Here's how the part is built. I have some questions about the finished solid (model axes, mm). A direction names the side the tool comes from. Coordinates: 2 decimals unless noted, no trailing zeros. Order: outer loops, then holes, each group sorted by start corner. A loop starts at its lowest first (then second) coordinate and runs counter-clockwise, first axis right, second up. Notation, with made-up numbers: (-17, -28.75) - (26, -28.75) arc R27 cw to (26, 1.25) - close; hole circle Ø6 at (-33.75, 17.25). An arc over 180 degrees is marked (long way). Answer as CSV lines item,"result". Start each with the question number.
Item 1: I'm going to push flat-ended pins straight in: pin 1 (2 mm diameter, centred on y = 12, z = 5, fed in from +X); pin 2 (4.5 mm diameter, centred on x = 19.5, z = 6, fed in from -Y); pin 3 (2 mm diameter, centred on x = 19, z = 4, fed in from +Y). Where does each tip first touch, or does it pass through?
Item 2: Imagine slicing it at D-D on x = -3. List the corners of the cut face in (y, z) for me, and give its area (3 significant figures).
Item 3: Imagine slicing it at A-A on x = 3. List the corners of the cut face in (y, z) for me, and give its area (3 significant figures).
Item 4: Imagine slicing it at C-C on z = 10.5. List the corners of the cut face in (x, y) for me, and give its area (3 significant figures).
Item 5: On a 3-axis mill with a long thin cutter (end or side, diameter ignored), from which of +Z, -Z, +X, -X, +Y, -Y can I reach the whole of each face in a straight line? I mean faces 1 (the face through (17, 8.069, 6)), 2 (the face through (-8, 10.569, 7)), 3 (the face through (-9, 9, 4.9)). Say none if no direction works.
Item 6: I need wall thicknesses on line 1 (Y direction, x = -2, z = 3); line 2 (X direction, y = 4, z = 7.25); line 3 (Y direction, x = -7.5, z = 1.75). Which ranges of each line are inside material? Lowest first, please.
Item 7: Imagine slicing it at B-B on y = 7. List the corners of the cut face in (x, z) for me, and give its area (4 significant figures).
from build123d import *

# Parameters (mm, degrees)
SKETCH2_W                = 22.5
SKETCH2_H                = 22.7
BOSS_EXTRUDE1_DEPTH      = 11.8
SKETCH3_R                = 5.9
BOSS_EXTRUDE2_DEPTH      = 4
SKETCH4_R                = 2.3
BOSS_EXTRUDE3_DEPTH      = 3.2
BOSS_EXTRUDE4_DEPTH      = 4
BOSS_EXTRUDE4_DEPTH_BACK = 26.5
SKETCH5_W                = 11.8
SKETCH5_H                = 2.5
CUT_EXTRUDE1_REACH       = 32.014


with BuildPart() as part:
    # Sketch2 → Boss-Extrude1 (new body)
    with BuildSketch(Plane.XY):
        with Locations((5.317300213, 3.518634424)):
            Rectangle(SKETCH2_W, SKETCH2_H)
    extrude(amount=BOSS_EXTRUDE1_DEPTH)

    # Sketch3 → Boss-Extrude2 (add)
    with BuildSketch(Plane(origin=(0, 14.868634424, 0), x_dir=(1, 0, 0), z_dir=(0, 1, 0))):
        with Locations((-0.032699787, -5.9)):
            Circle(SKETCH3_R)
        with BuildLine():
            ThreePointArc((5.31155509, -3.400212046), (5.726688366, -4.619590646), (5.867300213, -5.9))
            ThreePointArc((5.867300213, -5.9), (5.726688366, -7.180409354), (5.31155509, -8.399787954))
            ThreePointArc((5.31155509, -8.399787954), (7.844115569, -5.9), (5.31155509, -3.400212046))
        make_face()
    extrude(amount=BOSS_EXTRUDE2_DEPTH)

    # Sketch4 → Boss-Extrude3 (add)
    with BuildSketch(Plane(origin=(0, 18.868634424, 0), x_dir=(1, 0, 0), z_dir=(0, 1, 0))):
        with Locations(Location((-0.032699787, -5.9, 0), (0, 0, 270))):
            Circle(SKETCH4_R)
    extrude(amount=BOSS_EXTRUDE3_DEPTH)

    # Sketch5 → Boss-Extrude4 (add, two sides: drawn at the far end of the back side and taken through both)
    with BuildSketch(Plane(origin=(16.567300213, 0, 0), x_dir=(0, 0, -1), z_dir=(1, 0, 0)).offset(-BOSS_EXTRUDE4_DEPTH_BACK)):
        with Locations((-5.9, 9.318634424)):
            Rectangle(SKETCH5_W, SKETCH5_H)
    extrude(amount=BOSS_EXTRUDE4_DEPTH + BOSS_EXTRUDE4_DEPTH_BACK)

    # Sketch7 → Cut-Extrude1 (cut, up to next)
    with BuildSketch(Plane(origin=(0, 10.568634424, 0), x_dir=(1, 0, 0), z_dir=(0, 1, 0)), mode=Mode.PRIVATE) as cut_extrude1_sk1:
        with BuildLine():
            Line((20.567300213, -6.55), (20.567300213, -5.25))
            Line((20.567300213, -5.25), (19.027234421, -5.25))
            ThreePointArc((19.027234421, -5.25), (17.267300213, -5.9), (19.027234421, -6.55))
            Line((19.027234421, -6.55), (20.567300213, -6.55))
        make_face()
    cut_extrude1_tool1 = extrude(cut_extrude1_sk1.sketch, amount=-CUT_EXTRUDE1_REACH, mode=Mode.PRIVATE) & part.part
    # Sketch7 → Cut-Extrude1 (cut, up to next)
    with BuildSketch(Plane(origin=(0, 10.568634424, 0), x_dir=(1, 0, 0), z_dir=(0, 1, 0)), mode=Mode.PRIVATE) as cut_extrude1_sk2:
        with BuildLine():
            ThreePointArc((-8.392633994, -4.9), (-6.632699787, -5.55), (-8.392633994, -6.2))
            Line((-8.392633994, -6.2), (-9.932699787, -6.2))
            Line((-9.932699787, -6.2), (-9.932699787, -4.9))
            Line((-9.932699787, -4.9), (-8.392633994, -4.9))
        make_face()
    cut_extrude1_tool2 = extrude(cut_extrude1_sk2.sketch, amount=-CUT_EXTRUDE1_REACH, mode=Mode.PRIVATE) & part.part
    add(cut_extrude1_tool1.solids().sort_by_distance((18.851481, 10.568634, 5.9))[0], mode=Mode.SUBTRACT)
    add(cut_extrude1_tool2.solids().sort_by_distance((-8.216881, 10.568634, 5.55))[0], mode=Mode.SUBTRACT)


solid = part.part
Responses:
1,pin 1,"stops at x = 16.57"
1,pin 2,"stops at y = 8.07"
1,pin 3,"stops at y = 10.57"
2,outline,"(-7.83, 0) - (14.87, 0) - (14.87, 0.8) - (18.87, 0.8) - (18.87, 11) - (14.87, 11) - (14.87, 11.8) - (-7.83, 11.8) - close"
2,area,"309 mm^2"
3,outline,"(-7.83, 0) - (14.87, 0) - (14.87, 0.84) - (18.87, 0.84) - (18.87, 10.96) - (14.87, 10.96) - (14.87, 11.8) - (-7.83, 11.8) - close"
3,area,"308 mm^2"
4,outline,"(-9.93, 8.07) - (-5.93, 8.07) - (-5.93, -7.83) - (16.57, -7.83) - (16.57, 8.07) - (20.57, 8.07) - (20.57, 10.57) - (16.57, 10.57) - (16.57, 14.87) - (3.66, 14.87) - (3.66, 18.87) - (-3.73, 18.87) - (-3.73, 14.87) - (-5.93, 14.87) - (-5.93, 10.57) - (-9.93, 10.57) - close"
4,area,"560 mm^2"
5,face 1,"+Z, -Z, +X, -Y"
5,face 2,"+Z, -Z, -X, +Y"
5,face 3,"-X, +Y, -Y"
6,line 1,"y = -7.83 to 18.87"
6,line 2,"x = -5.93 to 16.57"
6,line 3,"y = 8.07 to 10.57"
7,outline,"(-5.93, 0) - (16.57, 0) - (16.57, 11.8) - (-5.93, 11.8) - close"
7,area,"265.5 mm^2"
